Could you check a few things on this model? Use its own coordinates, in mm. A direction names the side the tool comes from. Coordinates: 2 decimals unless noted, no trailing zeros. Loops run counter-clockwise (first coordinate to the right, second up) from the corner with the lowest first, then second, coordinate; pieces in that order, holes last. Notation, with made-up numbers: (-31, 86.25) - (14, 86.25) arc R20 cw to (14, 94.25) - close; hole circle Ø5 at (84, -30.75). An arc over 180 degrees is marked (long way). Use CSV: the item, a comma, the result in double quotes.
from build123d import *

# Parameters (mm, degrees)
ESQUISSE1_R             = 2
BOSS_EXTRU_1_DEPTH      = 5
CHANFREIN1_SIZE         = 1
ESQUISSE2_W             = 9
ESQUISSE2_H             = 50
ENL_V_MAT_EXTRU_1_DEPTH = 3


with BuildPart() as part:
    # Esquisse1 → Boss.-Extru.1 (new body)
    with BuildSketch(Plane(origin=(0, 0, 0), x_dir=(1, 0, 0), z_dir=(0, 1, 0))):
        with BuildLine():
            Line((-45, 25), (45, 25))
            ThreePointArc((45, 25), (47.121320344, 24.121320344), (48, 22))
            Line((48, 22), (48, -22))
            ThreePointArc((48, -22), (47.121320344, -24.121320344), (45, -25))
            Line((45, -25), (-45, -25))
            ThreePointArc((-45, -25), (-47.121320344, -24.121320344), (-48, -22))
            Line((-48, -22), (-48, 22))
            ThreePointArc((-48, 22), (-47.121320344, 24.121320344), (-45, 25))
        make_face()
        with Locations(Location((-43.5, 15, 0), (0, 0, 270))):
            Circle(ESQUISSE1_R, mode=Mode.SUBTRACT)
        with Locations(Location((43.5, 15, 0), (0, 0, 270))):
            Circle(ESQUISSE1_R, mode=Mode.SUBTRACT)
        with Locations(Location((43.5, -15, 0), (0, 0, 270))):
            Circle(ESQUISSE1_R, mode=Mode.SUBTRACT)
        with Locations(Location((-43.5, -15, 0), (0, 0, 270))):
            Circle(ESQUISSE1_R, mode=Mode.SUBTRACT)
    extrude(amount=-BOSS_EXTRU_1_DEPTH)

    # Chanfrein1
    chanfrein1_edges = [part.edges().sort_by_distance(p)[0] for p in [
        (-43.5, 0, -17),
        (43.5, 0, -17),
        (43.5, 0, 13),
        (-43.5, 0, 13),
    ]]
    chamfer(chanfrein1_edges, length=CHANFREIN1_SIZE)

    # Esquisse2 → Enlèv. mat.-Extru.1 (cut)
    with BuildSketch(Plane(origin=(0, -5, 0), x_dir=(-1, 0, 0), z_dir=(0, -1, 0))):
        with Locations((43.5, 0)):
            Rectangle(ESQUISSE2_W, ESQUISSE2_H)
        with Locations((-43.5, 0)):
            Rectangle(ESQUISSE2_W, ESQUISSE2_H)
    extrude(amount=-ENL_V_MAT_EXTRU_1_DEPTH, mode=Mode.SUBTRACT)


solid = part.part
(1) Which directions (+Z, -Z, +X, -X, +Y, -Y) give clear straight access to the entire face, cutting with the end or side of a thin tool? Please do faces 4 (the face through (-39, -4, 0)), 5 (the face through (-47.1, -0.99, 24.14)), 6 (the face through (44, -2, 0)).
Computed:
face 4,"+Z, -Z, -X, -Y"
face 5,"+Z, -X, +Y, -Y"
face 6,"+Z, -Z, +X, -Y"
(2) Thinking about a two-plate mould opening in X: for faces 1 (the face through (41.548, -1.493, 14.566)), 2 (the face through (-43, -2, 0)), 3 (the face through (-47.14, -0.99, -24.1)), which applies, +X half, -X half, draft (parallel to the pull), parting line (faces both ways), or undercut?
Computed:
face 1,"undercut"
face 2,"draft"
face 3,"-X half"
(3) Will these pins go through, and if not, where does the flat tip stop? pin 1 (4.5 mm diameter, centred on x = -42.5, z = 2.5, fed in from -Y); pin 2 (0.9 mm diameter, centred on y = -3, z = -4.5, fed in from -X).
Computed:
pin 1,"stops at y = -2"
pin 2,"stops at x = -39"
(4) Please list where these lines run through material, in increasing order: line 1 (X direction, y = -1.8, z = 15); line 2 (X direction, y = -2.8, z = -1.5); line 3 (Y direction, x = 42.5, z = -11).
Computed:
line 1,"x = -48 to -45.5, -41.5 to 41.5, 45.5 to 48"
line 2,"x = -39 to 39"
line 3,"y = -2 to 0"
(5) Suppose I cut it at A-A (z = 15). Write out the boundary of the cut face in (x, y), plus the area to 3 significant figures.
Computed:
outline,"(-48, -2) - (-45.5, -2) - (-45.5, -1) - (-46.5, 0) - (-48, 0) - close; (-41.5, -2) - (-39, -2) - (-39, -5) - (39, -5) - (39, -2) - (41.5, -2) - (41.5, -1) - (40.5, 0) - (-40.5, 0) - (-41.5, -1) - close; (45.5, -2) - (48, -2) - (48, 0) - (46.5, 0) - (45.5, -1) - close"
area,"408 mm²"
(6) Suppose I cut it at D-D (y = -2.9). Write out the boundary of the cut face in (x, z), plus the area to 3 significant figures.
Computed:
outline,"(-39, -25) - (39, -25) - (39, 25) - (-39, 25) - close"
area,"3,900 mm²"
(7) Suppose I cut it at C-C (z = 4.5). Write out the boundary of the cut face in (x, y), plus the area to 3 significant figures.
Computed:
outline,"(-48, -2) - (-39, -2) - (-39, -5) - (39, -5) - (39, -2) - (48, -2) - (48, 0) - (-48, 0) - close"
area,"426 mm²"
(8) Suppose I cut it at B-B (x = -43.5). Write out the boundary of the cut face in (y, z).
Computed:
outline,"(-2, -25) - (0, -25) - (0, -18) - (-1, -17) - (-2, -17) - close; (-2, -13) - (-1, -13) - (0, -12) - (0, 12) - (-1, 13) - (-2, 13) - close; (-2, 17) - (-1, 17) - (0, 18) - (0, 25) - (-2, 25) - close"
